Could you check a few things on this model? Use its own coordinates, in mm. Face numbers are marked on the shaded views. A direction names the side the tool comes from. Coordinates: 2 decimals unless noted, no trailing zeros. Order: outer loops, then holes, each group sorted by start corner. A loop starts at its lowest first (then second) coordinate and runs counter-clockwise, first axis right, second up.
```python
from build123d import *

# Parameters (mm, degrees)
SKETCH_W        = 80
SKETCH_H        = 65
PAD_DEPTH       = 4
SKETCH001_R     = 11.2
POCKET_DEPTH    = 4.001
SKETCH002_R     = 2
POCKET001_DEPTH = 4.001
SKETCH003_W     = 50.5
SKETCH003_H     = 48
SKETCH003_W_2   = 42.3
SKETCH003_H_2   = 42.3
PAD001_DEPTH    = 18
SKETCH004_R     = 3
POCKET002_DEPTH = 2
SKETCH005_R     = 2
POCKET003_DEPTH = 22.001
FILLET_R        = 10
FILLET001_R     = 2
CHAMFER_SIZE    = 2


with BuildPart() as part:
    # Sketch → Pad (new body)
    with BuildSketch(Plane.XY):
        with Locations((0, -7.5)):
            Rectangle(SKETCH_W, SKETCH_H)
    extrude(amount=PAD_DEPTH)

    # Sketch001 (on Face6 of Pad) → Pocket (cut, through all)
    with BuildSketch(Plane.XY.offset(4)):
        Circle(SKETCH001_R)
    extrude(amount=-POCKET_DEPTH, mode=Mode.SUBTRACT)

    # Sketch002 (on Face5 of Pocket) → Pocket001 (cut, through all)
    with BuildSketch(Plane.XY.offset(4)):
        with Locations((-15.5, 15.5)):
            Circle(SKETCH002_R)
        with Locations((-15.5, -15.5)):
            Circle(SKETCH002_R)
        with Locations((15.5, -15.5)):
            Circle(SKETCH002_R)
        with Locations((15.5, 15.5)):
            Circle(SKETCH002_R)
    extrude(amount=-POCKET001_DEPTH, mode=Mode.SUBTRACT)

    # Sketch003 (on Face4 of Pocket001) → Pad001 (join)
    with BuildSketch(Plane(origin=(0, 0, 0), x_dir=(1, 0, 0), z_dir=(0, 0, -1))):
        Rectangle(SKETCH003_W, SKETCH003_H)
        Rectangle(SKETCH003_W_2, SKETCH003_H_2, mode=Mode.SUBTRACT)
    extrude(amount=PAD001_DEPTH)

    # Sketch004 (on Face5 of Pad001) → Pocket002 (cut)
    with BuildSketch(Plane.XY.offset(4)):
        with Locations((-15.5, 15.5)):
            Circle(SKETCH004_R)
        with Locations((15.5, 15.5)):
            Circle(SKETCH004_R)
        with Locations((15.5, -15.5)):
            Circle(SKETCH004_R)
        with Locations((-15.5, -15.5)):
            Circle(SKETCH004_R)
    extrude(amount=-POCKET002_DEPTH, mode=Mode.SUBTRACT)

    # Sketch005 (on Face5 of Pocket002) → Pocket003 (cut, through all)
    with BuildSketch(Plane.XY.offset(4)):
        with Locations((-31.25, 16.25)):
            Circle(SKETCH005_R)
        with Locations((31.25, 16.25)):
            Circle(SKETCH005_R)
        with Locations((31.25, -31.25)):
            Circle(SKETCH005_R)
        with Locations((-31.25, -31.25)):
            Circle(SKETCH005_R)
    extrude(amount=-POCKET003_DEPTH, mode=Mode.SUBTRACT)

    # Fillet
    fillet_edges = [part.edges().sort_by_distance(p)[0] for p in [
        (40, -40, 2),
        (-40, -40, 2),
    ]]
    fillet(fillet_edges, radius=FILLET_R)

    # Fillet001
    fillet001_edges = [part.edges().sort_by_distance(p)[0] for p in [
        (25.25, -24, -9),
        (25.25, 24, -9),
        (-25.25, -24, -9),
        (-25.25, 24, -9),
    ]]
    fillet(fillet001_edges, radius=FILLET001_R)

    # Chamfer
    chamfer_edges = [part.edges().sort_by_distance(p)[0] for p in [
        (0, 25, 4),
        (-40, -2.5, 4),
    ]]
    chamfer(chamfer_edges, length=CHAMFER_SIZE)


solid = part.part
```
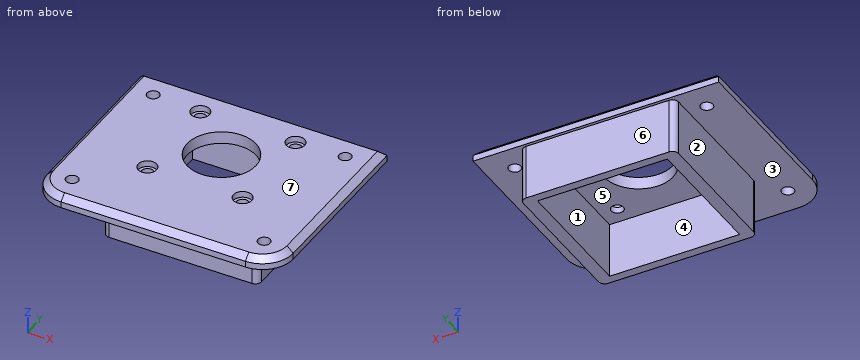
Item 1: Suppose I cut it at A-A (x = -15.5). Count the separate pieces of the cut face and the enclosed holes in it, and give its area (3 significant figures).
Item 2: Which directions (+Z, -Z, +X, -X, +Y, -Y) give clear straight access to the entire face, cutting with the end or side of a thin tool? Please do the marked faces 5, 6 and 7.
Item 3: Suppose I cut it at C-C (z = -5). List the corners of the cut face in (x, y) for me.
Item 4: For pin 1 Ø5.5 at (y, z) = (2.5, -11.5) entering from +X; pin 2 Ø10 at (x, z) = (-19.5, -5.5) entering from +Y; pin 3 Ø9 at (x, z) = (-4, -8.5) entering from -Y; pin 4 Ø3 at (x, y) = (-31.25, -31.25) entering from -Z, each with a flat end and sliding along its axis, tell me the tip position at first contact or that it passes through.
Item 5: Suppose I cut it at D-D (x = 7). List the corners of the cut face in (y, z) for me.
Item 6: I need wall thicknesses on line 1 (Y direction, x = 5.5, z = -9.75); line 2 (Y direction, x = 15.5, z = 0.9); line 3 (X direction, y = -9, z = -14.5). Which ranges of each line are inside material? Lowest first, please.
Item 7: Suppose I cut it at B-B (y = -1). List the corners of the cut face in (x, z) for me.
Item 8: Thinking about a two-plate mould opening in X: for the marked faces 1, 2, 3 and 4, which applies, +X half, -X half, draft (parallel to the pull), parting line (faces both ways), or undercut?
Geometry results:
1. separate pieces: 3
1. enclosed holes: 0
1. area: 319 mm2
2. face 5: -Z
2. face 6: -Z, +X, -X, +Y
2. face 7: +Z, +X, -X, +Y, -Y
3. outline: (-25.25, -22) arc R2 ccw to (-23.25, -24) - (23.25, -24) arc R2 ccw to (25.25, -22) - (25.25, 22) arc R2 ccw to (23.25, 24) - (-23.25, 24) arc R2 ccw to (-25.25, 22) - close; hole (-21.15, -21.15) - (21.15, -21.15) - (21.15, 21.15) - (-21.15, 21.15) - close
4. pin 1: stops at x = 25.25
4. pin 2: stops at y = 24
4. pin 3: stops at y = -24
4. pin 4: passes through
5. outline: (-40, 0) - (-24, 0) - (-24, -18) - (-21.15, -18) - (-21.15, 0) - (-8.74, 0) - (-8.74, 4) - (-38, 4) - (-40, 2) - close; (8.74, 0) - (21.15, 0) - (21.15, -18) - (24, -18) - (24, 0) - (25, 0) - (25, 2) - (23, 4) - (8.74, 4) - close
6. line 1: y = -24 to -21.15, 21.15 to 24
6. line 2: y = -40 to -17.5, -13.5 to 13.5, 17.5 to 25
6. line 3: x = -25.25 to -21.15, 21.15 to 25.25
7. outline: (-40, 0) - (-25.25, 0) - (-25.25, -18) - (-21.15, -18) - (-21.15, 0) - (-11.16, 0) - (-11.16, 4) - (-38, 4) - (-40, 2) - close; (11.16, 0) - (21.15, 0) - (21.15, -18) - (25.25, -18) - (25.25, 0) - (40, 0) - (40, 2) - (38, 4) - (11.16, 4) - close
8. face 1: undercut
8. face 2: -X half
8. face 3: draft
8. face 4: undercut
